```python
from build123d import *

# Parameters (mm, degrees)
BOSS_EXTRUDE1_DEPTH   = 10
FILLET1_R             = 2
FILLET2_R             = 2
F_4_0MM_DOWEL_HOLE1_D = 4


with BuildPart() as part:
    # Sketch1 → Boss-Extrude1 (new body)
    with BuildSketch(Plane(origin=(0, 0, 0), x_dir=(1, 0, 0), z_dir=(0, 1, 0))):
        with BuildLine():
            Line((-15, -2), (-5, -2))
            ThreePointArc((-5, -2), (0, -5.208712153), (5, -2))
            Line((5, -2), (15, -2))
            Line((15, -2), (15, 0))
            Line((15, 0), (5, 0))
            ThreePointArc((5, 0), (0, -3.208712153), (-5, 0))
            Line((-5, 0), (-15, 0))
            Line((-15, 0), (-15, -2))
        make_face()
    extrude(amount=BOSS_EXTRUDE1_DEPTH)

    # Fillet1
    fillet1_edges = [part.edges().sort_by_distance(p)[0] for p in [
        (5, 5, 2),
        (-5, 5, 2),
    ]]
    fillet(fillet1_edges, radius=FILLET1_R)

    # Fillet2
    fillet2_edges = [part.edges().sort_by_distance(p)[0] for p in [
        (15, 0, 1),
        (15, 10, 1),
        (-15, 10, 1),
        (-15, 0, 1),
    ]]
    fillet(fillet2_edges, radius=FILLET2_R)

    # Ø4.0mm Dowel Hole1 (through all)
    with Locations(Plane(origin=(0, 0, 0), x_dir=(1, 0, 0), z_dir=(0, 0, -1))):
        with Locations((10.5, -5), (-10.5, -5)):
            Hole(F_4_0MM_DOWEL_HOLE1_D / 2)


solid = part.part
```
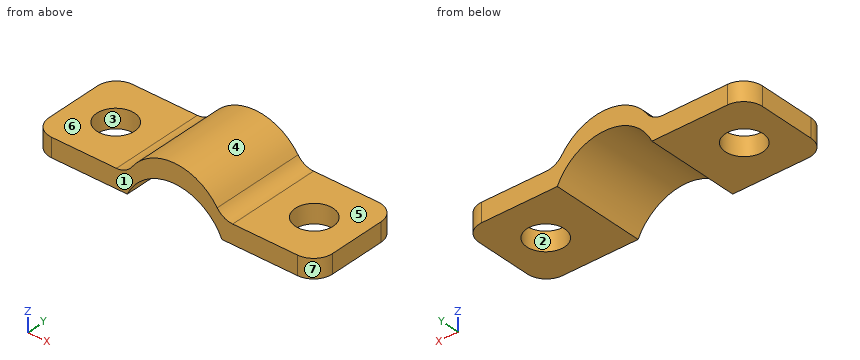
Read the model definition and answer for the solid it produces. Units are mm, in the model's axes. Face numbers are marked on the shaded views. A direction names the side the tool comes from. Coordinates: 2 decimals unless noted, no trailing zeros. Write each loop counter-clockwise with the first axis right and the second up, starting at its lowest first coordinate (ties: lowest second). Pieces come first, ordered by that corner, then holes. Notation, with made-up numbers: (42.5, -13) -> (62.5, -13) arc R24 ccw to (62.5, 25) -> close; hole circle Ø3 at (77, 36.25). An arc over 180 degrees is marked (long way). Return JSON: item names as keys, results as strings.
1. A cutting plane is placed at B-B (z = 1.2). Determine the outline of the cut face in (x, y), and give its area (3 significant figures).
Found:
{"outline": "(-15, 2) arc R2 ccw to (-13, 0) -> (-4.25, 0) -> (-4.25, 10) -> (-13, 10) arc R2 ccw to (-15, 8) -> close; (4.25, 0) -> (13, 0) arc R2 ccw to (15, 2) -> (15, 8) arc R2 ccw to (13, 10) -> (4.25, 10) -> close; hole circle Ø4 at (-10.5, 5); hole circle Ø4 at (10.5, 5)", "area": "186 mm2"}
2. A cutting plane is placed at D-D (y = 9.25). Determine the outline of the cut face in (x, z).
Found:
{"outline": "(-14.56, 0) -> (-5, 0) arc R5.5 cw to (5, 0) -> (14.56, 0) -> (14.56, 2) -> (6.15, 2) arc R2 cw to (4.51, 2.86) arc R5.5 ccw to (-4.51, 2.86) arc R2 cw to (-6.15, 2) -> (-14.56, 2) -> close"}
3. Determine the mould class of the marked faces 1, 2, 3 and 4 for opening direction Y: pulls with the +Y half, pulls with the -Y half, needs draft (parallel to the pull), parting line crosses it, or undercut.
Found:
{"face 1": "pulls with the -Y half", "face 2": "undercut", "face 3": "undercut", "face 4": "needs draft"}
4. A cutting plane is placed at C-C (x = 10.5). Determine the outline of the cut face in (y, z), and give its area (3 significant figures).
Found:
{"outline": "(0, 0) -> (3, 0) -> (3, 2) -> (0, 2) -> close; (7, 0) -> (10, 0) -> (10, 2) -> (7, 2) -> close", "area": "12.0 mm2"}
5. A tool of negligible diameter and unlimited length cuts with its end or side. For the marked faces 5, 6 and 7, from which of +Z, -Z, +X, -X, +Y, -Y can it reach the whole face along a straight path? Write none if from no direction.
Found:
{"face 5": "+Z, +X, +Y, -Y", "face 6": "+Z, -X, +Y, -Y", "face 7": "+Z, -Z, +X, -Y"}
6. Find the intervals of material crossed by line 1 along Y through (x, z) = (10.5, 1.35); line 2 along Z through (x, y) = (11, 2); line 3 along X through (y, z) = (0.5, 0.5), in increasing order. Write a range as from..to.
Found:
{"line 1": "0..3, 7..10", "line 2": "0..2", "line 3": "-14.32..-4.74, 4.74..14.32"}
7. A cutting plane is placed at A-A (y = 5). Determine the outline of the cut face in (x, z).
Found:
{"outline": "(-15, 0) -> (-12.5, 0) -> (-12.5, 2) -> (-15, 2) -> close; (-8.5, 0) -> (-5, 0) arc R5.5 cw to (5, 0) -> (8.5, 0) -> (8.5, 2) -> (6.15, 2) arc R2 cw to (4.51, 2.86) arc R5.5 ccw to (-4.51, 2.86) arc R2 cw to (-6.15, 2) -> (-8.5, 2) -> close; (12.5, 0) -> (15, 0) -> (15, 2) -> (12.5, 2) -> close"}
8. This flat-tipped pin is pushed along its axis until it touches: P1, Ø3, axis at y = 8.5, z = 4, coming from the +X side. Where does it stop, or does it pass through?
Found:
{"P1": "x = 4.83"}
